Here's how the part is built. I have some questions about the finished solid (model axes, mm). A direction names the side the tool comes from. Round coordinates to 2 decimals unless told otherwise and drop trailing zeros. Order: outer loops, then holes, each group sorted by start corner. A loop starts at its lowest first (then second) coordinate and runs counter-clockwise, first axis right, second up. Notation, with made-up numbers: M 81,-6.5 L 138,-6.5 A31 ccw 138,18.5 Z; hole C 41,68.5 d2. An arc over 180 degrees is marked long. Write item = value, one per line. Start each with the question number.
Item 1: I want a section at D-D, the plane z = -16. List the corners of the cut face in (x, y) for me, plus the area to 3 significant figures.
Item 2: We'd pull the mould along Y, two halves only. Please class faces 4 (the face through (2, -34.603, 36)), 5 (the face through (2, -56, -12)), 6 (the face through (1.97, -11.81, 22.15)): pulls with the +Y half, pulls with the -Y half, needs draft (parallel to the pull), parting line crosses it, or undercut.
Item 3: For faces 1 (the face through (2, -29, 34)), 2 (the face through (2, -56, 0)), 3 (the face through (2, 87.5, -37)), which set-ups out of +Z, -Z, +X, -X, +Y, -Y let a thin tool reach every point of the face, with its end or its side?
Item 4: I want a section at C-C, the plane z = 21. List the corners of the cut face in (x, y) for me, plus the area to 3 significant figures.
Item 5: Please list where these lines run through material, in increasing order: L1, parallel to Y at x = 1.6, z = -27; L2, parallel to Y at x = 3.15, z = 19; L3, parallel to Z at x = 3.65, y = 57.
Item 6: I want a section at B-B, the plane y = -10.5. List the corners of the cut face in (x, z) for me, plus the area to 3 significant figures.
Item 7: I'm going to push flat-ended pins straight in: P1, Ø1, axis at y = -34.5, z = 1, coming from the -X side; P2, Ø1, axis at x = 0.5, z = -25.5, coming from the +Y side. Where does each tip first touch, or does it pass through?
Item 8: I want a section at A-A, the plane x = 2.5. List the corners of the cut face in (y, z) for me, plus the area to 3 significant figures.
```python
from build123d import *

# Parameters (mm, degrees)
BOSS_EXTRUDE1_DEPTH = 4
CUT_EXTRUDE1_REACH  = 99.14
SKETCH3_R           = 3.41
CUT_EXTRUDE2_REACH  = 99.14
SKETCH4_R           = 3.41
CUT_EXTRUDE4_REACH  = 99.14


with BuildPart() as part:
    # Sketch1 → Boss-Extrude1 (new body)
    with BuildSketch(Plane(origin=(0, 0, 0), x_dir=(0, 0, -1), z_dir=(1, 0, 0))):
        Polygon((-38, -57.5), (42, -57.5), (42, 87.5), (32, 87.5), (-34, -23.740343039), (-34, -34.602813771), (-38, -34.602813771), align=None)
    extrude(amount=BOSS_EXTRUDE1_DEPTH)

    # Sketch3 → Cut-Extrude1 (cut, up to next)
    with BuildSketch(Plane.ZY, mode=Mode.PRIVATE) as cut_extrude1_sk1:
        with Locations((-27, -10.5)):
            Circle(SKETCH3_R)
    cut_extrude1_tool1 = extrude(cut_extrude1_sk1.sketch, amount=-CUT_EXTRUDE1_REACH, mode=Mode.PRIVATE) & part.part
    # Sketch3 → Cut-Extrude1 (cut, up to next)
    with BuildSketch(Plane.ZY, mode=Mode.PRIVATE) as cut_extrude1_sk2:
        with Locations((19, -10.5)):
            Circle(SKETCH3_R)
    cut_extrude1_tool2 = extrude(cut_extrude1_sk2.sketch, amount=-CUT_EXTRUDE1_REACH, mode=Mode.PRIVATE) & part.part
    add(cut_extrude1_tool1.solids().sort_by_distance((0, -10.5, -27))[0], mode=Mode.SUBTRACT)
    add(cut_extrude1_tool2.solids().sort_by_distance((0, -10.5, 19))[0], mode=Mode.SUBTRACT)

    # Sketch4 → Cut-Extrude2 (cut, up to next)
    with BuildSketch(Plane.ZY, mode=Mode.PRIVATE) as cut_extrude2_sk1:
        with Locations((-27, -47.5)):
            Circle(SKETCH4_R)
    cut_extrude2_tool1 = extrude(cut_extrude2_sk1.sketch, amount=-CUT_EXTRUDE2_REACH, mode=Mode.PRIVATE) & part.part
    # Sketch4 → Cut-Extrude2 (cut, up to next)
    with BuildSketch(Plane.ZY, mode=Mode.PRIVATE) as cut_extrude2_sk2:
        with Locations((19, -47.5)):
            Circle(SKETCH4_R)
    cut_extrude2_tool2 = extrude(cut_extrude2_sk2.sketch, amount=-CUT_EXTRUDE2_REACH, mode=Mode.PRIVATE) & part.part
    add(cut_extrude2_tool1.solids().sort_by_distance((0, -47.5, -27))[0], mode=Mode.SUBTRACT)
    add(cut_extrude2_tool2.solids().sort_by_distance((0, -47.5, 19))[0], mode=Mode.SUBTRACT)

    # Sketch6 → Cut-Extrude4 (cut, up to next)
    with BuildSketch(Plane(origin=(4, 0, 0), x_dir=(0, 0, -1), z_dir=(1, 0, 0)), mode=Mode.PRIVATE) as cut_extrude4_sk1:
        with BuildLine():
            Line((0, -54.5), (0, -57.5))
            Line((0, -57.5), (12, -57.5))
            Line((12, -57.5), (12, -54.5))
            ThreePointArc((12, -54.5), (6, -48.5), (0, -54.5))
        make_face()
    cut_extrude4_tool1 = extrude(cut_extrude4_sk1.sketch, amount=-CUT_EXTRUDE4_REACH, mode=Mode.PRIVATE) & part.part
    add(cut_extrude4_tool1.solids().sort_by_distance((4, -53.527539, -6))[0], mode=Mode.SUBTRACT)


solid = part.part
```
Filled in:
q1.outline = M 0,-57.5 L 4,-57.5 L 4,60.53 L 0,60.53 Z
q1.area = 472 mm^2
q2.face_4 = pulls with the +Y half
q2.face_5 = needs draft
q2.face_6 = undercut
q3.face_1 = +Z, +X, -X, +Y
q3.face_2 = +X, -X, -Y
q3.face_3 = +Z, -Z, +X, -X, +Y
q4.outline = M 0,-57.5 L 4,-57.5 L 4,-50.26 L 0,-50.26 Z; M 0,-44.74 L 4,-44.74 L 4,-13.26 L 0,-13.26 Z; M 0,-7.74 L 4,-7.74 L 4,-1.83 L 0,-1.83 Z
q4.area = 178 mm^2
q5.L1 = -57.5 to -50.91, -44.09 to -13.91, -7.09 to 79.07
q5.L2 = -57.5 to -50.91, -44.09 to -13.91, -7.09 to 1.54
q5.L3 = -42 to -13.9
q6.outline = M 0,-42 L 4,-42 L 4,-30.41 L 0,-30.41 Z; M 0,-23.59 L 4,-23.59 L 4,15.59 L 0,15.59 Z; M 0,22.41 L 4,22.41 L 4,26.14 L 0,26.14 Z
q6.area = 218 mm^2
q7.P1 = 0
q7.P2 = 77.39
q8.outline = M -57.5,-42 L 87.5,-42 L 87.5,-32 L -23.74,34 L -34.6,34 L -34.6,38 L -57.5,38 L -57.5,0 L -54.5,0 A6 cw -54.5,-12 L -57.5,-12 Z; hole C -47.5,-27 d6.82; hole C -47.5,19 d6.82; hole C -10.5,-27 d6.82; hole C -10.5,19 d6.82
q8.area = 7,200 mm^2
